Source: CAD feature listing. Evaluate the final solid. Frame: model axes, mm. Give positions to 0.01 mm unless a question says otherwise; leave off trailing zeros. Order: outer loops, then holes, each group sorted by start corner. A loop starts at its lowest first (then second) coordinate and runs counter-clockwise, first axis right, second up. Notation, with made-up numbers: M 7.25,53.5 L 39.25,53.5 A8 cw 39.25,58.5 Z; hole C 19.5,86.25 d5. An arc over 180 degrees is marked long. Return JSON: item names as keys, results as strings.
from build123d import *

# Parameters (mm, degrees)
F0_W     = 550
F0_H     = 44
F1_DEPTH = 1.5
F2_W     = 10
F2_H     = 14
F3_DEPTH = 3
F4_R     = 1.5
F5_DEPTH = 15


with BuildPart() as f1:
    # F0 (on Front) → F1 (new body)
    with BuildSketch(Plane.XZ):
        with Locations((275, 22)):
            Rectangle(F0_W, F0_H)
    extrude(amount=F1_DEPTH)

    # F2 (on face) → F3 (join)
    with BuildSketch(Plane.XZ.offset(1.5)):
        with Locations((5, 22)):
            Rectangle(F2_W, F2_H)
    extrude(amount=F3_DEPTH)

    # F4 (on face) → F5 (join)
    with BuildSketch(Plane(origin=(0, 0, 0), x_dir=(0, -1, 0), z_dir=(-1, 0, 0))):
        with Locations((2.5, 25.5)):
            Circle(F4_R)
        with Locations((2.5, 18.5)):
            Circle(F4_R)
    extrude(amount=F5_DEPTH)


solid = f1.part
1. Section query A-A (y = -2.5). Return loops of the section in (x, z), then the cut area to 3 significant figures.
Evaluation:
{"outline": "M -15,17 L 0,17 L 0,15 L 10,15 L 10,29 L 0,29 L 0,27 L -15,27 L -15,24 L 0,24 L 0,20 L -15,20 Z", "area": "230 mm^2"}
2. Section query B-B (x = 456.5). Return loops of the section in (y, z), then the cut area to 3 significant figures.
Evaluation:
{"outline": "M -1.5,0 L 0,0 L 0,44 L -1.5,44 Z", "area": "66.0 mm^2"}
3. First-contact query: pin 1 (1.5 mm diameter, centred on x = 7.5, y = -3, fed in from +Z); pin 2 (0.9 mm diameter, centred on x = 6, y = -3.5, fed in from -Z); pin 3 (22 mm diameter, centred on x = 347, z = 16.5, fed in from -Y). Flat tips, straight axial feed; report the tip coordinate or a pass-through.
Evaluation:
{"pin 1": "stops at z = 29", "pin 2": "stops at z = 15", "pin 3": "stops at y = -1.5"}
4. Ray query, probe 1 along Y at (x, z) = (107.5, 3); probe 2 along X at (y, z) = (-0.25, 15.5); probe 3 along X at (y, z) = (-3.4, 22). Return the intervals inside material, ascending.
Evaluation:
{"probe 1": "y = -1.5 to 0", "probe 2": "x = 0 to 550", "probe 3": "x = 0 to 10"}
